The model under review builds one solid part; all positions refer to its coordinate system, in mm. A direction names the side the tool comes from. Round coordinates to 2 decimals unless told otherwise and drop trailing zeros. Order: outer loops, then holes, each group sorted by start corner. A loop starts at its lowest first (then second) coordinate and runs counter-clockwise, first axis right, second up. Notation, with made-up numbers: M 70,20.5 L 75,20.5 A10 ccw 75,27.5 Z; hole C 29,51.5 d7. An arc over 180 degrees is marked long. Use a Markdown table: item, result. Add a question column.
1. For faces 4 (the flat face through (-5, 336.55, 826)), 5 (the flat face through (-5, -322, 25.4)), 6 (the flat face through (5, -380, 1168.4)), 7 (the flat face through (-4, -179.07, 759)), 8 (the flat face through (-2, -336.55, 1669)), list the 3-axis set-ups (+Z, -Z, +X, -X, +Y, -Y) from which the entire face can be reached by the end or side of a thin tool; tool diameter is ignored.
2. The part is to be moulded in two halves that separate along Z. For faces 1 (the flat face through (-355.6, -322, 827)), 2 (the flat face through (-5, 20, 1676.4)), 3 (the flat face through (-5, -380, 1193.8)), say which applies: +Z half, -Z half, draft (parallel to the pull), parting line (faces both ways), or undercut.
3. Consider section B-B on x = 93.5. State the section outline as (y, z) points.
4. Consider section C-C on y = -130.5. State the section outline as (x, z) points.
5. Insertion check: P1, Ø24.5, axis at y = -323, z = 665, coming from the +X side; P2, Ø5, axis at x = 13.5, y = -57.5, coming from the -Z side; P3, Ø15, axis at y = -324.5, z = 743, coming from the -X side. Each pin has a flat end and moves straight along its axis. Give the tip position at first contact, or say it passes through.
6. Consider section A-A on z = 762.5. State the section outline as (x, y) points, then the cut area to 3 significant figures.
7. To check wall thickness, follow probe 1 along X at (y, z) = (108, 739); probe 2 along Y at (x, z) = (-79, 577); probe 3 along Z at (x, y) = (166.5, -355.5). State the ranges of each line that lie inside material, in increasing order.
from build123d import *

# Parameters (mm, degrees)
F0_W     = 762
F0_H     = 673.1
F1_DEPTH = 1676.4
F2_W     = 762
F2_H     = 1676.4
F2_W_2   = 711.2
F2_H_2   = 1625.6
F3_DEPTH = 30.48
F4_W     = 711.2
F4_H     = 457.2
F4_W_2   = 25.4
F4_H_2   = 1066.8
F5_DEPTH = 88.9
F6_W     = 508
F6_H     = 388.62
F7_DEPTH = 1539.24


with BuildPart() as f1:
    # F0 (on Top) → F1 (new body)
    with BuildSketch(Plane.XY):
        Rectangle(F0_W, F0_H)
    extrude(amount=F1_DEPTH)

    # F2 (on face) → F3 (cut)
    with BuildSketch(Plane.XZ.offset(336.55)):
        with Locations((0, 838.2)):
            Rectangle(F2_W, F2_H)
        with Locations((0, 838.2)):
            Rectangle(F2_W_2, F2_H_2, mode=Mode.SUBTRACT)
    extrude(amount=-F3_DEPTH, mode=Mode.SUBTRACT)

    # F4 (on face) → F5 (join)
    with BuildSketch(Plane.XZ.offset(336.55)):
        with Locations((0, 1422.4)):
            Rectangle(F4_W, F4_H)
        Polygon((381, 1676.4), (-381, 1676.4), (-381, 1193.8), (-355.6, 1193.8), (-355.6, 1651), (355.6, 1651), (355.6, 1193.8), (381, 1193.8), align=None)
        with Locations((368.3, 635)):
            Rectangle(F4_W_2, F4_H_2)
        with Locations((0, 635)):
            Rectangle(F4_W, F4_H_2)
        with Locations((-368.3, 635)):
            Rectangle(F4_W_2, F4_H_2)
    extrude(amount=F5_DEPTH)

    # F6 (on face) → F7 (cut)
    with BuildSketch(Plane(origin=(0, 0, 0), x_dir=(1, 0, 0), z_dir=(0, 0, -1))):
        with Locations((0, -15.24)):
            Rectangle(F6_W, F6_H)
    extrude(amount=-F7_DEPTH, mode=Mode.SUBTRACT)


solid = f1.part
Answer block:
| question | item | result |
|---|---|---|
| 1 | face 4 | +Z, -Z, +X, -X, +Y |
| 1 | face 5 | -Z, +X, -X, -Y |
| 1 | face 6 | +X, -X, -Y |
| 1 | face 7 | -Z |
| 1 | face 8 | +Z |
| 2 | face 1 | draft |
| 2 | face 2 | +Z half |
| 2 | face 3 | undercut |
| 3 | outline | M -425.45,101.6 L -336.55,101.6 L -336.55,25.4 L -306.07,25.4 L -306.07,0 L -179.07,0 L -179.07,1539.24 L 209.55,1539.24 L 209.55,0 L 336.55,0 L 336.55,1676.4 L -306.07,1676.4 L -306.07,1651 L -336.55,1651 L -336.55,1676.4 L -425.45,1676.4 L -425.45,1193.8 L -336.55,1193.8 L -336.55,1168.4 L -425.45,1168.4 Z |
| 4 | outline | M -381,0 L -254,0 L -254,1539.24 L 254,1539.24 L 254,0 L 381,0 L 381,1676.4 L -381,1676.4 Z |
| 5 | P1 | x = 355.6 |
| 5 | P2 | z = 1539.24 |
| 5 | P3 | x = -355.6 |
| 6 | outline | M -381,-425.45 L 381,-425.45 L 381,-336.55 L 355.6,-336.55 L 355.6,-306.07 L 381,-306.07 L 381,336.55 L -381,336.55 L -381,-306.07 L -355.6,-306.07 L -355.6,-336.55 L -381,-336.55 Z; hole M -254,-179.07 L 254,-179.07 L 254,209.55 L -254,209.55 Z |
| 6 | area | 382,000 mm^2 |
| 7 | probe 1 | -381 to -254, 254 to 381 |
| 7 | probe 2 | -425.45 to -179.07, 209.55 to 336.55 |
| 7 | probe 3 | 101.6 to 1168.4, 1193.8 to 1676.4 |
